```python
from build123d import *

# Parameters (mm, degrees)
SKETCH_1_W          = 30.5
SKETCH_1_H          = 12
EXTRUDE_1_DEPTH     = 18
SKETCH_2_W          = 30.5
SKETCH_2_H          = 12
CUT_EXTRUDE_2_DEPTH = 6.2
SKETCH_3_R          = 2
SKETCH_3_W          = 4
SKETCH_3_H          = 1
CUT_EXTRUDE_3_DEPTH = 11.5
CUT_EXTRUDE_4_DEPTH = 8
SKETCH_5_W          = 3.964363922
SKETCH_5_H          = 1
CUT_EXTRUDE_6_DEPTH = 7
SKETCH_6_W          = 3.964363922
SKETCH_6_H          = 6
CUT_EXTRUDE_7_DEPTH = 26.822712871
FILLET_1_R          = 2
FILLET_2_R          = 2
FILLET_3_R          = 1
SKETCH_7_W          = 17.4
SKETCH_7_H          = 5.750693342
CUT_EXTRUDE_8_DEPTH = 10.5
SKETCH_9_OUTSIDE_W  = 39.978
SKETCH_9_OUTSIDE_H  = 21.478
SKETCH_9_OUTSIDE_R  = 0.5
CUT_EXTRUDE_9_DEPTH = 6.1
SKETCH_8_R          = 0.25
EXTRUDE_2_DEPTH     = 3


with BuildPart() as part:
    # 草图1 → 凸台-拉伸1 (new body)
    with BuildSketch(Plane(origin=(0, 0, 0), x_dir=(1, 0, 0), z_dir=(0, 1, 0))):
        Rectangle(SKETCH_1_W, SKETCH_1_H)
    extrude(amount=EXTRUDE_1_DEPTH)

    # 草图2 → 切除-拉伸2 (cut)
    with BuildSketch(Plane(origin=(0, 18, 0), x_dir=(1, 0, 0), z_dir=(0, 1, 0))):
        Rectangle(SKETCH_2_W, SKETCH_2_H)
        with BuildLine():
            Line((-6.556600226, 3), (6.556600226, 3))
            ThreePointArc((6.556600226, 3), (6.924541369, 2.838554744), (7.054873105, 2.45847726))
            Line((7.054873105, 2.45847726), (6.638206438, -2.54152274))
            ThreePointArc((6.638206438, -2.54152274), (6.478488304, -2.867941143), (6.139933559, -3))
            Line((6.139933559, -3), (-6.139933559, -3))
            ThreePointArc((-6.139933559, -3), (-6.478488304, -2.867941143), (-6.638206438, -2.54152274))
            Line((-6.638206438, -2.54152274), (-7.054873105, 2.45847726))
            ThreePointArc((-7.054873105, 2.45847726), (-6.924541369, 2.838554744), (-6.556600226, 3))
        make_face(mode=Mode.SUBTRACT)
    extrude(amount=-CUT_EXTRUDE_2_DEPTH, mode=Mode.SUBTRACT)

    # 草图3 → 切除-拉伸3 (cut)
    with BuildSketch(Plane(origin=(0, 11.8, 0), x_dir=(1, 0, 0), z_dir=(0, 1, 0))):
        with Locations(Location((12.25, 0, 0), (0, 0, 270))):
            Circle(SKETCH_3_R)
        with Locations(Location((-12.25, 0, 0), (0, 0, 90))):
            Circle(SKETCH_3_R)
        with Locations((12.25, -5.5)):
            Rectangle(SKETCH_3_W, SKETCH_3_H)
        with Locations((-12.25, -5.5)):
            Rectangle(SKETCH_3_W, SKETCH_3_H)
    extrude(amount=-CUT_EXTRUDE_3_DEPTH, mode=Mode.SUBTRACT)

    # 草图4 → 切除-拉伸4 (cut)
    with BuildSketch(Plane.XZ):
        Polygon((8.5, -4.6), (8.5, 3.5), (15.25, 3.5), (15.25, -4.6), (15.25, -6), (-15.25, -6), (-15.25, 3.5), (-8.5, 3.5), (-8.5, -4.6), align=None)
    extrude(amount=-CUT_EXTRUDE_4_DEPTH, mode=Mode.SUBTRACT)

    # 草图5 → 切除-拉伸6 (cut)
    with BuildSketch(Plane.XZ):
        with Locations((12.267818039, 4)):
            Rectangle(SKETCH_5_W, SKETCH_5_H)
        with Locations((-12.267818039, 4)):
            Rectangle(SKETCH_5_W, SKETCH_5_H)
    extrude(amount=-CUT_EXTRUDE_6_DEPTH, mode=Mode.SUBTRACT)

    # 草图6 → 切除-拉伸7 (cut, through all)
    with BuildSketch(Plane(origin=(0, 0, 4.5), x_dir=(-1, 0, 0), z_dir=(0, 0, -1))):
        with Locations((12.267818039, 4)):
            Rectangle(SKETCH_6_W, SKETCH_6_H)
    cut_extrude_7 = extrude(amount=-CUT_EXTRUDE_7_DEPTH, mode=Mode.SUBTRACT)

    # 圆角1
    # the kernel refuses this fillet: 2 mm, written as the material it adds along each edge
    with BuildSketch(Plane(origin=(-14.25, 1, 4.5), x_dir=(0, 1, 0), z_dir=(0, 0, 1)), Plane(origin=(-10.285636078, 1, 4.5), x_dir=(-1, 0, 0), z_dir=(0, 0, 1))) as fillet_1_piece_1:
        with BuildLine():
            CenterArc((FILLET_1_R, -FILLET_1_R), FILLET_1_R, 90, 90)
            Line((0, -FILLET_1_R), (0, 0))
            Line((0, 0), (FILLET_1_R, 0))
        make_face()
    extrude(amount=0.5)
    with BuildSketch(Plane(origin=(-14.25, 7, 3.5), x_dir=(0, -1, 0), z_dir=(0, 0, 1))) as fillet_1_piece_2:
        with BuildLine():
            CenterArc((FILLET_1_R, FILLET_1_R), FILLET_1_R, 180, 90)
            Line((0, FILLET_1_R), (0, 0))
            Line((0, 0), (FILLET_1_R, 0))
        make_face()
    extrude(amount=1.5)
    with BuildSketch(Plane(origin=(-10.285636078, 7, 3.5), x_dir=(0, -1, 0), z_dir=(0, 0, 1))) as fillet_1_piece_3:
        with BuildLine():
            CenterArc((FILLET_1_R, -FILLET_1_R), FILLET_1_R, 90, 90)
            Line((0, -FILLET_1_R), (0, 0))
            Line((0, 0), (FILLET_1_R, 0))
        make_face()
    extrude(amount=1.5)

    # 镜向1: 切除-拉伸7 across plane
    add(cut_extrude_7.mirror(Plane(origin=(0, 0, 0), x_dir=(0, 0, 1), z_dir=(1, 0, 0))), mode=Mode.SUBTRACT)

    # 圆角2
    # the kernel refuses this fillet: 2 mm, written as the material it adds along each edge
    with BuildSketch(Plane(origin=(14.25, 1, 4.5), x_dir=(-1, 0, 0), z_dir=(0, 0, 1))) as fillet_2_piece_1:
        with BuildLine():
            CenterArc((FILLET_2_R, -FILLET_2_R), FILLET_2_R, 90, 90)
            Line((0, -FILLET_2_R), (0, 0))
            Line((0, 0), (FILLET_2_R, 0))
        make_face()
    extrude(amount=0.5)
    with BuildSketch(Plane(origin=(10.285636078, 1, 4.5), x_dir=(1, 0, 0), z_dir=(0, 0, 1))) as fillet_2_piece_2:
        with BuildLine():
            CenterArc((FILLET_2_R, FILLET_2_R), FILLET_2_R, 180, 90)
            Line((0, FILLET_2_R), (0, 0))
            Line((0, 0), (FILLET_2_R, 0))
        make_face()
    extrude(amount=0.5)
    with BuildSketch(Plane(origin=(10.285636078, 7, 3.5), x_dir=(1, 0, 0), z_dir=(0, 0, 1)), Plane(origin=(14.25, 7, 5), x_dir=(-1, 0, 0), z_dir=(0, 0, -1))) as fillet_2_piece_3:
        with BuildLine():
            CenterArc((FILLET_2_R, -FILLET_2_R), FILLET_2_R, 90, 90)
            Line((0, -FILLET_2_R), (0, 0))
            Line((0, 0), (FILLET_2_R, 0))
        make_face()
    extrude(amount=1.5)

    # 圆角3
    fillet_3_edges = [part.edges().sort_by_distance(p)[0] for p in [
        (-15.25, 9.9, -6),
        (15.25, 9.9, -6),
        (-8.5, 4, -4.6),
        (8.5, 4, -4.6),
    ]]
    fillet(fillet_3_edges, radius=FILLET_3_R)

    # 草图7 → 切除-拉伸8 (cut)
    with BuildSketch(Plane.XZ):
        with Locations((0, 7.875346671)):
            Rectangle(SKETCH_7_W, SKETCH_7_H)
    extrude(amount=-CUT_EXTRUDE_8_DEPTH, mode=Mode.SUBTRACT)

    # 草图9 outside → 切除-拉伸9 (cut)
    with BuildSketch(Plane(origin=(0, 18, 0), x_dir=(1, 0, 0), z_dir=(0, 1, 0))):
        Rectangle(SKETCH_9_OUTSIDE_W, SKETCH_9_OUTSIDE_H)
        with Locations(Location((0, 1.27, 0), (0, 0, 270))):
            Circle(SKETCH_9_OUTSIDE_R, mode=Mode.SUBTRACT)
        with Locations(Location((2.54, 1.27, 0), (0, 0, 270))):
            Circle(SKETCH_9_OUTSIDE_R, mode=Mode.SUBTRACT)
        with Locations(Location((5.08, 1.27, 0), (0, 0, 270))):
            Circle(SKETCH_9_OUTSIDE_R, mode=Mode.SUBTRACT)
        with Locations(Location((-5.08, 1.27, 0), (0, 0, 90))):
            Circle(SKETCH_9_OUTSIDE_R, mode=Mode.SUBTRACT)
        with Locations(Location((-2.54, 1.27, 0), (0, 0, 90))):
            Circle(SKETCH_9_OUTSIDE_R, mode=Mode.SUBTRACT)
        with Locations(Location((-1.27, -1.27, 0), (0, 0, 270))):
            Circle(SKETCH_9_OUTSIDE_R, mode=Mode.SUBTRACT)
        with Locations(Location((-3.81, -1.27, 0), (0, 0, 270))):
            Circle(SKETCH_9_OUTSIDE_R, mode=Mode.SUBTRACT)
        with Locations(Location((3.81, -1.27, 0), (0, 0, 90))):
            Circle(SKETCH_9_OUTSIDE_R, mode=Mode.SUBTRACT)
        with Locations(Location((1.27, -1.27, 0), (0, 0, 90))):
            Circle(SKETCH_9_OUTSIDE_R, mode=Mode.SUBTRACT)
    extrude(amount=-CUT_EXTRUDE_9_DEPTH, mode=Mode.SUBTRACT)

    # 草图8 → 凸台-拉伸2 (add)
    with BuildSketch(Plane.XY.offset(5)):
        with Locations(Location((0, 1.27, 0), (0, 0, 180))):
            Circle(SKETCH_8_R)
        with Locations(Location((2.77, 1.27, 0), (0, 0, 180))):
            Circle(SKETCH_8_R)
        with Locations(Location((5.54, 1.27, 0), (0, 0, 180))):
            Circle(SKETCH_8_R)
        with Locations(Location((-5.54, 1.27, 0), (0, 0, 180))):
            Circle(SKETCH_8_R)
        with Locations(Location((-2.77, 1.27, 0), (0, 0, 180))):
            Circle(SKETCH_8_R)
        with Locations(Location((-1.385, 4.11, 0), (0, 0, 180))):
            Circle(SKETCH_8_R)
        with Locations(Location((1.385, 4.11, 0), (0, 0, 180))):
            Circle(SKETCH_8_R)
        with Locations(Location((-4.155, 4.11, 0), (0, 0, 180))):
            Circle(SKETCH_8_R)
        with Locations(Location((4.155, 4.11, 0), (0, 0, 180))):
            Circle(SKETCH_8_R)
    extrude(amount=EXTRUDE_2_DEPTH)


solid = part.part
```
Check sheet for the modelled part. Datum: model origin and axes. Units: mm. A direction names the side the tool comes from. Round coordinates to 2 decimals unless told otherwise and drop trailing zeros. Write each loop counter-clockwise with the first axis right and the second up, starting at its lowest first coordinate (ties: lowest second). Pieces come first, ordered by that corner, then holes. Notation, with made-up numbers: M -30.5,83 L -6.5,83 A20 ccw -6.5,121 Z; hole C 22,-24.75 d1. An arc over 180 degrees is marked long. Write item = value, one per line. Start each with the question number.
1. Release check for a two-part mould opening along X. For faces 6 (the flat face through (8.5, 4, 0)), 7 (the cylindrical face through (10.88, 6.42, 4.24)), 8 (the flat face through (-8.5, 4, 0)) record: pulls with the +X half, pulls with the -X half, needs draft (parallel to the pull), parting line crosses it, or undercut.
2. Section check C-C, the plane z = 0. Record the cut outline in (x, y).
3. Section check A-A, the plane y = 15.75. State how many separate pieces and enclosed holes the cut face has, then the cut area to 3 significant figures.
4. Section check D-D, the plane y = 8.5. Record the cut outline in (x, z).
5. Gauge pin test, flat ends, axial feed: pin 1 (5 mm diameter, centred on y = 16, z = 2.5, fed in from +X); pin 2 (4.5 mm diameter, centred on x = -13, y = 4, fed in from +Z); pin 3 (0.8 mm diameter, centred on x = 12.5, z = 5.5, fed in from +Y). Record the tip position at first contact, or that the pin passes through.
6. Tool access check on faces 1 (the flat face through (12.3, 7.4, 5)), 2 (the flat face through (-8.7, 5.2, 5.5)), 3 (the cylindrical face through (-8.215, 4.056, -4.299)), 4 (the cylindrical face through (1.1, 15, 0.8)), 5 (the flat face through (-14.25, 4.5, 5)). Record the directions out of +Z, -Z, +X, -X, +Y, -Y that give a thin tool (end or side, any length) a straight path to the whole face; none if there is none.
7. Scan lines: line 1 (X direction, y = 10, z = 0); line 2 (X direction, y = 15.5, z = 1.5); line 3 (Y direction, x = 12, z = 5.5). Record each from-to range of solid material in increasing order. Write a range as [from, to].
Results found:
q1.face_6 = pulls with the +X half
q1.face_7 = undercut
q1.face_8 = pulls with the -X half
q2.outline = M -15.25,8 L -14.25,8 L -14.25,11.8 L -15.25,11.8 Z; M -10.25,8 L -8.5,8 L -8.5,0 L 8.5,0 L 8.5,8 L 10.25,8 L 10.25,11.8 L 6.85,11.8 L 6.85,11.9 L -6.85,11.9 L -6.85,11.8 L -10.25,11.8 Z; M 14.25,8 L 15.25,8 L 15.25,11.8 L 14.25,11.8 Z
q3.separate_pieces = 9
q3.enclosed_holes = 0
q3.area = 7.07 mm^2
q4.outline = M -15.25,-5 A1 ccw -14.25,-6 L 14.25,-6 A1 ccw 15.25,-5 L 15.25,6 L 14.25,6 L 14.25,5 L 10.25,5 L 10.25,6 L 8.7,6 L 8.7,5 L -8.7,5 L -8.7,6 L -10.25,6 L -10.25,5 L -14.25,5 L -14.25,6 L -15.25,6 Z; hole C -12.25,0 d4; hole C 12.25,0 d4
q5.pin_1 = 4.31
q5.pin_2 = 6
q5.pin_3 = 0.3
q6.face_1 = +Z, +Y
q6.face_2 = +Z, -Y
q6.face_3 = -Z, -X, -Y
q6.face_4 = +Y
q6.face_5 = none
q7.line_1 = [-15.25, -14.25], [-10.25, 10.25], [14.25, 15.25]
q7.line_2 = [-4.25, -3.37], [-1.71, -0.83], [0.83, 1.71], [3.37, 4.25]
q7.line_3 = [0, 0.3]
